The listing builds one solid part. Answer for the finished solid, in the listing's coordinates (mm). A direction names the side the tool comes from. Round coordinates to 2 decimals unless told otherwise and drop trailing zeros. Loops run counter-clockwise (first coordinate to the right, second up) from the corner with the lowest first, then second, coordinate; pieces in that order, holes last. Notation, with made-up numbers: (-17, 43) - (15, 43) arc R13 cw to (15, 68) - close; hole circle Ø7 at (16, 22). An arc over 180 degrees is marked (long way). One line per item, written item: value.
```python
from build123d import *

# Parameters (mm, degrees)
F0_R     = 3.048
F0_W     = 19.05
F0_H     = 3.302
F1_DEPTH = 13.97
F2_R     = 2.54
F3_R     = 3.048
F4_DEPTH = 3.302
F5_DEPTH = 13.97


with BuildPart() as f1:
    # F0 (on Top) → F1 (new body)
    with BuildSketch(Plane.XY):
        Polygon((9.525, 6.223), (-9.525, 6.223), (-9.525, -9.525), (-3.175, -9.525), (9.525, -9.525), align=None)
        Circle(F0_R, mode=Mode.SUBTRACT)
        with Locations((0, 7.874)):
            Rectangle(F0_W, F0_H)
    extrude(amount=F1_DEPTH)

    # F2
    f2_edges = [f1.edges().sort_by_distance(p)[0] for p in [
        (9.525, 9.525, 6.985),
        (-9.525, 9.525, 6.985),
        (9.525, -9.525, 6.985),
    ]]
    fillet(f2_edges, radius=F2_R)

    # F3 (on face) → F4 (join)
    with BuildSketch(Plane.XY.offset(13.97)):
        Circle(F3_R)
    extrude(amount=-F4_DEPTH)

    # F0 (on Top) → F5 (join, through all)
    with BuildSketch(Plane.XY):
        with BuildLine():
            Line((-3.175, -9.525), (-9.525, -9.525))
            Line((-9.525, -9.525), (-9.525, -20.955))
            ThreePointArc((-9.525, -20.955), (-6.35, -24.13), (-3.175, -20.955))
            Line((-3.175, -20.955), (-3.175, -9.525))
        make_face()
    extrude(amount=F5_DEPTH)


solid = f1.part
```
1) A cutting plane is placed at B-B on x = 0. Give the vertices of the cut face in (y, z) (3 decimals).
Final values:
outline: (-9.525, 0) - (-3.048, 0) - (-3.048, 10.668) - (3.048, 10.668) - (3.048, 0) - (9.525, 0) - (9.525, 13.97) - (-9.525, 13.97) - close
2) A cutting plane is placed at C-C on z = 11.75. Give the vertices of the cut face in (x, y) (3 decimals).
Final values:
outline: (-9.525, -20.955) arc R3.175 ccw to (-3.175, -20.955) - (-3.175, -9.525) - (6.985, -9.525) arc R2.54 ccw to (9.525, -6.985) - (9.525, 6.985) arc R2.54 ccw to (6.985, 9.525) - (-6.985, 9.525) arc R2.54 ccw to (-9.525, 6.985) - close
3) For a pull along Y with two mould halves and no side action, classify faces 4 (the flat face through (0, 9.525, 7)), 5 (the flat face through (0, 0, 10.668)), 6 (the flat face through (-2, -3, 0)) as released by +Y, released by -Y, zero draft, split by the parting line, or undercut.
Final values:
face 4: released by +Y
face 5: undercut
face 6: zero draft
4) For faces 1 (the cylindrical face through (-0.4, 3.02, 5.26)), 2 (the cylindrical face through (-6.42, -24.13, 6.89)), 3 (the flat face through (2, -9.525, 7)), determine the directions among +Z, -Z, +X, -X, +Y, -Y from which every point of the face is accessible in a straight line to the end or side of a thin tool.
Final values:
face 1: -Z
face 2: +Z, -Z, -Y
face 3: +Z, -Z, +X, -Y
5) This flat-tipped pin is pushed along its axis until it touches: pin 1 Ø8 at (x, z) = (2, 3.5) entering from -Y (3 decimals). Where does it stop, or does it pass through?
Final values:
pin 1: y = -9.525
6) A cutting plane is placed at A-A on z = 7.75. Give the vertices of the cut face in (x, y) (3 decimals).
Final values:
outline: (-9.525, -20.955) arc R3.175 ccw to (-3.175, -20.955) - (-3.175, -9.525) - (6.985, -9.525) arc R2.54 ccw to (9.525, -6.985) - (9.525, 6.985) arc R2.54 ccw to (6.985, 9.525) - (-6.985, 9.525) arc R2.54 ccw to (-9.525, 6.985) - close; hole circle Ø6.096 at (0, 0)
7) Consider L1, parallel to Y at x = 0, z = 3.5 (3 decimals); L2, parallel to Y at x = -1.75, z = 11 (3 decimals); L3, parallel to X at y = -1.5, z = 5.5 (3 decimals). Determine where each line is inside the solid, lowest interval first.
Final values:
L1: -9.525 to -3.048, 3.048 to 9.525
L2: -9.525 to 9.525
L3: -9.525 to -2.653, 2.653 to 9.525
